from build123d import *

# Parameters (mm, degrees)
F2_R     = 38
F3_DEPTH = 95


with BuildPart() as f1:
    # F0 (on Front) → F1 (revolve)
    with BuildSketch(Plane.XZ):
        with BuildLine():
            Line((5.073e-07, 40.0000000001), (-1e-10, 0))
            Line((0, 0), (7.5000005075, -7e-10))
            Line((7.5000005075, -7e-10), (7.5000005075, 42.0000000001))
            ThreePointArc((7.5000005075, 42.0000000001), (6.9142140698, 40.5857864377), (5.5000005075, 40.0000000001))
            Line((5.5000005075, 40.0000000001), (5.073e-07, 40.0000000001))
        make_face()
        Polygon((7.5000005075, 42.0000000001), (7.5000005075, -7e-10), (9.0000005075, -9e-10), (9.0000005075, 59.9999999993), (7.5000005075, 59.9999999993), align=None)
        Polygon((9.0000005075, 59.9999999993), (9.0000005075, -9e-10), (98.5000005577, -9.5e-09), (98.5000005577, 43.954244746), (98.5000005577, 44.218735217), align=None)
    revolve(axis=Axis((46.8394961208, 0, 0), (1, 0, 0)))

    # F2 (on face) → F3 (cut)
    with BuildSketch(Plane(origin=(2.536e-07, 0, 0), x_dir=(0, -1, 0), z_dir=(-1, 0, 0))):
        Circle(F2_R)
    extrude(amount=-F3_DEPTH, mode=Mode.SUBTRACT)


solid = f1.part
Could you check a few things on this model? Use its own coordinates, in mm. A direction names the side the tool comes from. Round coordinates to 2 decimals unless told otherwise and drop trailing zeros. Loops run counter-clockwise (first coordinate to the right, second up) from the corner with the lowest first, then second, coordinate; pieces in that order, holes last. Notation, with made-up numbers: (6.5, 70.5) - (61.5, 70.5) arc R7 cw to (61.5, 82.5) - close; hole circle Ø6 at (48, -17). An arc over 180 degrees is marked (long way). Write item = value, one per line.
1) Imagine slicing it at A-A (x = 29). Please give me the cut outline in (y, z), and give its area (3 significant figures).
Computed:
outline = circle Ø112.95 at (0, 0); hole circle Ø76 at (0, 0)
area = 5,480 mm2
2) Imagine slicing it at B-B (x = 12.5). Please give me the cut outline in (y, z), and give its area (3 significant figures).
Computed:
outline = circle Ø118.77 at (0, 0); hole circle Ø76 at (0, 0)
area = 6,540 mm2
3) I need wall thicknesses on line 1 along X through (y, z) = (16.5, 38.5); line 2 along X through (y, z) = (2.5, -12.5); line 3 along Y through (x, z) = (24, 19.5). Which ranges of each line are inside material? Lowest first, please. Write a range as from..to.
Computed:
line_1 = 7.5..98.5
line_2 = 95..98.5
line_3 = -53.94..-32.62, 32.62..53.94
4) I'm going to push flat-ended pins straight in: P1, Ø2, axis at x = 72.5, y = 39.5, coming from the -Z side; P2, Ø4, axis at x = 67, z = -47, coming from the -Y side; P3, Ø6, axis at x = 47, y = -37, coming from the -Z side. Where does each tip first touch, or does it pass through?
Computed:
P1 = -30.02
P2 = -21.35
P3 = -41.14
5) If we mould it in two halves opening along Y, with no side actions, what happens to faces 3 (the flat face through (95, 1, 1)), 4 (the flat face through (98.5, -1, 1)), 5 (the conical face through (63.068, -42.553, 27.13))? For each: pulls with the +Y half, pulls with the -Y half, needs draft (parallel to the pull), parting line crosses it, or undercut.
Computed:
face_3 = undercut
face_4 = needs draft
face_5 = parting line crosses it
6) On a 3-axis mill with a long thin cutter (end or side, diameter ignored), from which of +Z, -Z, +X, -X, +Y, -Y can I reach the whole of each face in a straight line? I mean faces 1 (the flat face through (7.5, 12, -41)), 2 (the cylindrical face through (8.24, 58.573, -13.007)). Say none if no direction works.
Computed:
face_1 = -X
face_2 = +X, -X
